Can you work these out from the model? Positions are in its coordinate system, mm. A direction names the side the tool comes from. Round coordinates to 2 decimals unless told otherwise and drop trailing zeros. Write each loop counter-clockwise with the first axis right and the second up, starting at its lowest first coordinate (ties: lowest second). Pieces come first, ordered by that corner, then holes.
Q1. If we section it at B-B (z = 46): Please give me the cut outline in (x, y), plus the area to 3 significant figures.
Q2. For faces 1 (the cylindrical face through (-6.738, -6.37, 1.479)), 2 (the flat face through (-7, 5, 3)), which set-ups out of +Z, -Z, +X, -X, +Y, -Y let a thin tool reach every point of the face, with its end or its side?
Q3. If we section it at A-A (z = 14.5): Please give me the cut outline in (x, y), plus the area to 3 significant figures.
Q4. Please list where these lines run through material, in increasing order: line 1 along Y through (x, z) = (-6, 13.5); line 2 along Z through (x, y) = (8, 5); line 3 along X through (y, z) = (1.25, 37.5).
Q5. I'm going to push flat-ended pins straight in: pin 1 Ø4 at (x, y) = (7.99, 6.42) entering from +Z; pin 2 Ø6 at (y, z) = (-6.5, 27.5) entering from -X; pin 3 Ø5 at (x, z) = (3.5, 11.5) entering from -Y. Where does each tip first touch, or does it pass through?
Q6. If we section it at C-C (z = 20.5): Please give me the cut outline in (x, y), plus the area to 3 significant figures.
Q7. We'd pull the mould along X, two halves only. Please class faces 3 (the cylindrical face through (-6.937, -10.399, 1.651)), 4 (the flat face through (-8, -8, 3)), 5 (the flat face through (0, 0, 0)): +X half, -X half, draft (parallel to the pull), parting line (faces both ways), or undercut.
from build123d import *

# Parameters (mm, degrees)
F0_R           = 1.25
F1_DEPTH       = 5
F3_D           = 2.5
F3_DEPTH       = 5
F3_CBORE_D     = 4.4
F3_CBORE_DEPTH = 2
F3_TIP         = 0.7510757738
F4_DEPTH       = 45


# Not quite as in the source:
# - a fillet or chamfer that OpenCascade refuses, or shapes differently, is made with other operations: its cross-section is extruded or revolved along the edge and cut away or added


with BuildPart() as f1:
    # F0 (on Top) → F1 (new body)
    with BuildSketch(Plane.XY):
        with BuildLine():
            ThreePointArc((9.7397717911, -7.8349757789), (11.7897656336, -4.1534836349), (12.5, 0))
            ThreePointArc((12.5, 0), (11.7897656358, 4.1534836287), (9.7397717994, 7.8349757687))
            ThreePointArc((9.7397717994, 7.8349757687), (6.6e-09, 12.5), (-9.7397717911, 7.8349757789))
            ThreePointArc((-9.7397717911, 7.8349757789), (-12.5, 0), (-9.7397717911, -7.8349757789))
            ThreePointArc((-9.7397717911, -7.8349757789), (0, -12.5), (9.7397717911, -7.8349757789))
        make_face()
        with BuildLine():
            ThreePointArc((-5.7366128015, -6.4246802223), (-7.2389857978, -8.5468380541), (-9.7397717911, -7.8349757789))
            ThreePointArc((-9.7397717911, -7.8349757789), (-8.7342398052, -4.3025223904), (-5.7366128015, -6.4246802223))
        make_face(mode=Mode.SUBTRACT)
        with BuildLine():
            ThreePointArc((10.2366128015, -6.4246802223), (10.1087706334, -7.172307226), (9.7397717911, -7.8349757789))
            ThreePointArc((9.7397717911, -7.8349757789), (5.8644549697, -5.6770532186), (10.2366128015, -6.4246802223))
        make_face(mode=Mode.SUBTRACT)
        with BuildLine():
            ThreePointArc((-5.7366128015, 6.4246802223), (-8.7342398052, 4.3025223904), (-9.7397717911, 7.8349757789))
            ThreePointArc((-9.7397717911, 7.8349757789), (-7.2389857978, 8.5468380541), (-5.7366128015, 6.4246802223))
        make_face(mode=Mode.SUBTRACT)
        with BuildLine():
            ThreePointArc((10.2366128015, 6.4246802223), (5.8644549675, 5.6770532248), (9.7397717994, 7.8349757687))
            ThreePointArc((9.7397717994, 7.8349757687), (10.1087706356, 7.1723072198), (10.2366128015, 6.4246802223))
        make_face(mode=Mode.SUBTRACT)
        with BuildLine():
            ThreePointArc((10.2366128015, 6.4246802223), (10.1087706356, 7.1723072198), (9.7397717994, 7.8349757687))
            ThreePointArc((9.7397717994, 7.8349757687), (5.8644549675, 5.6770532248), (10.2366128015, 6.4246802223))
        make_face()
        with Locations((7.9866128015, 6.4246802223)):
            Circle(F0_R, mode=Mode.SUBTRACT)
        with BuildLine():
            ThreePointArc((10.2366128015, -6.4246802223), (5.8644549697, -5.6770532186), (9.7397717911, -7.8349757789))
            ThreePointArc((9.7397717911, -7.8349757789), (10.1087706334, -7.172307226), (10.2366128015, -6.4246802223))
        make_face()
        with Locations((7.9866128015, -6.4246802223)):
            Circle(F0_R, mode=Mode.SUBTRACT)
        with BuildLine():
            ThreePointArc((-5.7366128015, -6.4246802223), (-8.7342398052, -4.3025223904), (-9.7397717911, -7.8349757789))
            ThreePointArc((-9.7397717911, -7.8349757789), (-7.2389857978, -8.5468380541), (-5.7366128015, -6.4246802223))
        make_face()
        with Locations((-7.9866128015, -6.4246802223)):
            Circle(F0_R, mode=Mode.SUBTRACT)
        with BuildLine():
            ThreePointArc((-5.7366128015, 6.4246802223), (-7.2389857978, 8.5468380541), (-9.7397717911, 7.8349757789))
            ThreePointArc((-9.7397717911, 7.8349757789), (-8.7342398052, 4.3025223904), (-5.7366128015, 6.4246802223))
        make_face()
        with Locations((-7.9866128015, 6.4246802223)):
            Circle(F0_R, mode=Mode.SUBTRACT)
        with Locations((7.9866128015, 6.4246802223)):
            Circle(F0_R)
        with Locations((7.9866128015, -6.4246802223)):
            Circle(F0_R)
        with Locations((-7.9866128015, -6.4246802223)):
            Circle(F0_R)
        with Locations((-7.9866128015, 6.4246802223)):
            Circle(F0_R)
    extrude(amount=F1_DEPTH)

    # F3
    with Locations(Plane.XY.offset(5)):
        with Locations((-7.9866128015, 6.4246802223), (-7.9866128015, -6.4246802223), (7.9866128015, -6.4246802223), (7.9866128015, 6.4246802223)):
            CounterBoreHole(F3_D / 2, F3_CBORE_D / 2, F3_CBORE_DEPTH, depth=F3_DEPTH)
            with Locations((0, 0, -(F3_DEPTH + F3_TIP / 2))):  # 118° drill point
                Cone(0, F3_D / 2, F3_TIP, mode=Mode.SUBTRACT)

    # F4 (add): a face of the model
    f4_faces = [f1.faces().sort_by_distance(p)[0] for p in [
        (0, 0, 5),
    ]]
    extrude(f4_faces, amount=F4_DEPTH)

    # F5: chamfer of 12.5 x 46.6506350946 on 1 edges, made by hand

    # F5_s1 → F5_t2 (revolve, cut)
    with BuildSketch(Plane(origin=(0, 0, 0), x_dir=(0, 0, 1), z_dir=(0.6267980623, 0.7791817433, 0))):
        Polygon((3.3493649054, -12.5), (50, 0), (50, -12.5), align=None)
    revolve(axis=Axis((0, 0, 50), (0, 0, 1)), mode=Mode.SUBTRACT)


solid = f1.part
A:
1. outline: circle Ø2.14 at (0, 0)
1. area: 3.61 mm2
2. face 1: +Z, -Z
2. face 2: +Z
3. outline: (-8.49, -4.28) arc R2.2 cw to (-6, -7.38) arc R9.51 ccw to (6, -7.38) arc R2.2 cw to (8.49, -4.28) arc R9.51 ccw to (8.49, 4.28) arc R2.2 cw to (6, 7.38) arc R9.51 ccw to (-6, 7.38) arc R2.2 cw to (-8.49, 4.28) arc R9.51 ccw to start
3. area: 268 mm2
4. line 1: y = -7.72 to -7.37, -5.48 to 5.48, 7.37 to 7.72
4. line 2: z = 0 to 3
4. line 3: x = -3.11 to 3.11
5. pin 1: stops at z = 3
5. pin 2: stops at x = -5.12
5. pin 3: stops at y = -10.67
6. outline: circle Ø15.81 at (0, 0)
6. area: 196 mm2
7. face 3: parting line
7. face 4: undercut
7. face 5: draft
